Study the drawing (mm; zero at the part's minimum x, y, z) and answer. A direction names the side the tool comes from. Round coordinates to 2 decimals unless told otherwise and drop trailing zeros. Loops run counter-clockwise (first coordinate to the right, second up) from the corner with the lowest first, then second, coordinate; pieces in that order, holes last. Notation, with made-up numbers: M 51.25,-24.5 L 61.25,-24.5 A30 cw 61.25,9.5 Z; hole C 10.5,-18.5 d6. An arc over 180 degrees is marked long. Write each question's results on one line, items separated by ' | '.
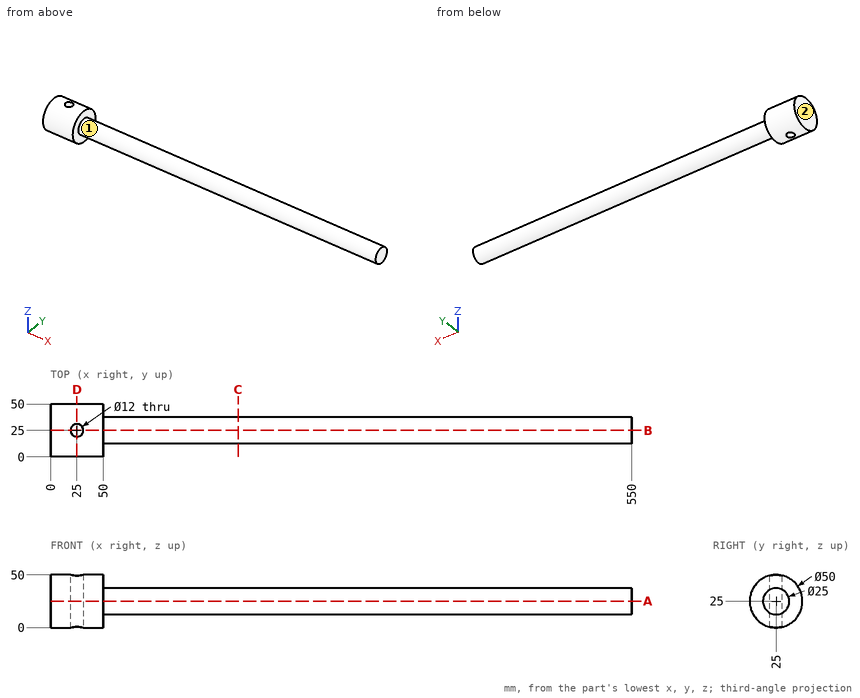
Item 1: The part is cut by section D-D (x = 25). Determine the outline of the cut face in (y, z).
Outcome:
outline: M 19,0.73 L 19,49.27 A25 ccw Z; M 31,0.73 A25 ccw 31,49.27 Z
Item 2: Flat-ended cylindrical pins translate along their axes: pin 1 (4 mm diameter, centred on x = 371.5, z = 35.5, fed in from +Y); pin 2 (6 mm diameter, centred on x = 367, z = 33.5, fed in from +Y) (3 decimals); pin 3 (1 mm diameter, centred on x = 400, y = 22, fed in from +Z). Find the tip coordinate at first contact, or state that the pin passes through.
Outcome:
pin 1: stops at y = 34.17 | pin 2: stops at y = 36.225 | pin 3: stops at z = 37.25
Item 3: The part is cut by section B-B (y = 25). Determine the outline of the cut face in (x, z), plus the area to 3 significant figures.
Outcome:
outline: M 0,0 L 19,0 L 19,50 L 0,50 Z; M 31,0 L 50,0 L 50,12.5 L 550,12.5 L 550,37.5 L 50,37.5 L 50,50 L 31,50 Z | area: 14,400 mm2
Item 4: The part is cut by section C-C (x = 177.5). Determine the outline of the cut face in (y, z).
Outcome:
outline: C 25,25 d25
Item 5: For the marked faces 1 and 2, determine the directions among +Z, -Z, +X, -X, +Y, -Y from which every point of the face is accessible in a straight line to the end or side of a thin tool.
Outcome:
face 1: +X | face 2: +Z, -Z, -X, +Y, -Y
Item 6: The part is cut by section A-A (z = 25). Determine the outline of the cut face in (x, y).
Outcome:
outline: M 0,0 L 50,0 L 50,12.5 L 550,12.5 L 550,37.5 L 50,37.5 L 50,50 L 0,50 Z; hole C 25,25 d12
Item 7: Straight lines are drawn through the part: line 1 (X direction, y = 24.5, z = 30); line 2 (X direction, y = 36, z = 39); line 3 (Y direction, x = 84.5, z = 36). For each, find the intervals that lie inside material, in ascending order.
Outcome:
line 1: x = 0 to 19.02, 30.98 to 550 | line 2: x = 0 to 50 | line 3: y = 19.06 to 30.94
